```python
from build123d import *

# Parameters (mm, degrees)
EXTRUDE_1_DEPTH          = 5
CHAMFER_1_SIZE           = 10
CUT_EXTRUDE_1_DEPTH      = 61.279402969
CUT_EXTRUDE_1_DEPTH_BACK = 61.279402969
SKETCH_2_R               = 2.1
EXTRUDE_START            = 37
SKETCH_3_W               = 10
SKETCH_3_H               = 14.142135624
SKETCH_3_R               = 2.1
EXTRUDE_2_DEPTH          = 37
SKETCH_4_W               = 10
SKETCH_4_H               = 20
EXTRUDE_3_DEPTH          = 6
SKETCH_6_W               = 10
SKETCH_6_H               = 32
EXTRUDE_5_DEPTH          = 6
CUT_EXTRUDE_2_DEPTH      = 15
CUT_EXTRUDE_3_DEPTH      = 72.219678224
SKETCH_10_W              = 15
SKETCH_10_H              = 3.8
EXTRUDE_6_DEPTH          = 3
CHAMFER_2_SIZE           = 2
CHAMFER_3_SIZE           = 2
CHAMFER_4_SIZE           = 5
CHAMFER_5_SIZE           = 2
SKETCH_12_R              = 3.2
CUT_EXTRUDE_4_DEPTH      = 38
CUT_EXTRUDE_5_DEPTH      = 4


with BuildPart() as part:
    # 草图1 → 凸台-拉伸1 (new, symmetric)
    with BuildSketch(Plane.XY):
        Polygon((-10, 0), (33.5, 43.5), (38.5, 38.5), (0, 0), (38.5, -38.5), (33.5, -43.5), align=None)
    extrude(amount=EXTRUDE_1_DEPTH, both=True)

    # 倒角1
    chamfer_1_edges = [part.edges().sort_by_distance(p)[0] for p in [
        (-10, 0, 0),
        (0, 0, 0),
    ]]
    chamfer(chamfer_1_edges, length=CHAMFER_1_SIZE)

    # 草图2 → 切除-拉伸1 (cut, two sides: drawn at the far end of the back side and taken through both)
    with BuildSketch(Plane.ZY.offset(2.928932188).offset(-CUT_EXTRUDE_1_DEPTH_BACK)):
        with Locations(Location((0, 0, 0), (0, 0, 270))):
            Circle(SKETCH_2_R)
    extrude(amount=CUT_EXTRUDE_1_DEPTH + CUT_EXTRUDE_1_DEPTH_BACK, mode=Mode.SUBTRACT)

    # 草图3 → 凸台-拉伸2 (add)
    with BuildSketch(Plane.ZY.offset(2.928932188).offset(EXTRUDE_START)):
        Rectangle(SKETCH_3_W, SKETCH_3_H)
        with Locations(Location((0, 0, 0), (0, 0, 270))):
            Circle(SKETCH_3_R, mode=Mode.SUBTRACT)
    extrude(amount=-EXTRUDE_2_DEPTH)

    # 草图4 → 凸台-拉伸3 (add)
    with BuildSketch(Plane(origin=(38.5, 38.5, 0), x_dir=(0, 0, -1), z_dir=(0.7071067811865467, 0.7071067811865485, 0))):
        with Locations((-10, -2.928932188)):
            Rectangle(SKETCH_4_W, SKETCH_4_H)
    extrude_3 = extrude(amount=-EXTRUDE_3_DEPTH)

    # 草图6 → 凸台-拉伸5 (add)
    with BuildSketch(Plane(origin=(38.5, 38.5, 0), x_dir=(0, 0, -1), z_dir=(0.7071067811865467, 0.7071067811865485, 0))):
        with Locations((-10, 3.071067812)):
            Rectangle(SKETCH_6_W, SKETCH_6_H)
    extrude_5 = extrude(amount=-EXTRUDE_5_DEPTH)

    # 草图8 → 切除-拉伸2 (cut)
    with BuildSketch(Plane.XY.offset(15)):
        Polygon((21.549895398, 48.520458146), (44.177312396, 25.893041148), (46.864318164, 28.580046917), (24.236901166, 51.207463915), align=None)
    cut_extrude_2 = extrude(amount=-CUT_EXTRUDE_2_DEPTH, mode=Mode.SUBTRACT)

    # 草图9 → 切除-拉伸3 (cut, through all)
    with BuildSketch(Plane(origin=(0, 0, 5), x_dir=(-1, 0, 0), z_dir=(0, 0, -1))):
        Polygon((-32.722182541, 42.722182541), (-24.236901166, 51.207463915), (-25.014718626, 51.985281374), (-33.5, 43.5), align=None)
        Polygon((-21.549895398, 48.520458146), (-30.035176772, 40.035176772), (-29.257359313, 39.257359313), (-20.772077939, 47.742640687), align=None)
    cut_extrude_3 = extrude(amount=-CUT_EXTRUDE_3_DEPTH, mode=Mode.SUBTRACT)

    # 草图10 → 凸台-拉伸6 (add)
    with BuildSketch(Plane(origin=(-5, 5, 0), x_dir=(0, 0, 1), z_dir=(-0.7071067811865487, 0.7071067811865465, 0))):
        with Locations((7.5, 51.447222151)):
            Rectangle(SKETCH_10_W, SKETCH_10_H)
    extrude_6 = extrude(amount=-EXTRUDE_6_DEPTH)

    # 倒角2
    chamfer_2_edges = [part.edges().sort_by_distance(p)[0] for p in [
        (47.253226894, 28.968955647, 15),
        (31.378679656, 41.378679656, 15),
        (22.785533906, 22.785533906, -5),
        (43.788403666, 25.504132419, 5),
        (43.788403666, 25.504132419, 15),
        (15.285533906, 25.285533906, -5),
        (38.11109127, 38.11109127, 5),
        (47.253226894, 28.968955647, 5),
    ]]
    chamfer(chamfer_2_edges, length=CHAMFER_2_SIZE)

    # 镜向1: 凸台-拉伸3, 凸台-拉伸5, 切除-拉伸2, 切除-拉伸3, 凸台-拉伸6 across plane
    add(extrude_3.mirror(Plane.ZX))
    add(extrude_5.mirror(Plane.ZX))
    add(cut_extrude_2.mirror(Plane.ZX), mode=Mode.SUBTRACT)
    add(cut_extrude_3.mirror(Plane.ZX), mode=Mode.SUBTRACT)
    add(extrude_6.mirror(Plane.ZX))

    # 倒角3
    chamfer_3_edges = [part.edges().sort_by_distance(p)[0] for p in [
        (38.11109127, -38.11109127, 5),
        (15.285533906, -25.285533906, -5),
        (43.788403666, -25.504132419, 5),
        (43.788403666, -25.504132419, 15),
        (34.646268043, -34.646268043, 5),
        (47.253226894, -28.968955647, 5),
        (47.253226894, -28.968955647, 15),
        (31.378679656, -41.378679656, 15),
        (22.785533906, -22.785533906, -5),
    ]]
    chamfer(chamfer_3_edges, length=CHAMFER_3_SIZE)

    # 倒角4
    chamfer_4_edges = [part.edges().sort_by_distance(p)[0] for p in [
        (31.757359313, -36.757359313, 5),
        (31.757359313, 36.757359313, 5),
    ]]
    chamfer(chamfer_4_edges, length=CHAMFER_4_SIZE)

    # 倒角5
    chamfer_5_edges = [part.edges().sort_by_distance(p)[0] for p in [
        (-20.014718626, -7.071067812, -5),
        (-20.014718626, 7.071067812, -5),
        (-21.428932188, -7.071067812, 5),
        (-21.428932188, 7.071067812, 5),
    ]]
    chamfer(chamfer_5_edges, length=CHAMFER_5_SIZE)

    # 草图12 → 切除-拉伸4 (cut)
    with BuildSketch(Plane.ZY.offset(39.928932188)):
        with Locations(Location((0, 0, 0), (0, 0, 270))):
            Circle(SKETCH_12_R)
    extrude(amount=-CUT_EXTRUDE_4_DEPTH, mode=Mode.SUBTRACT)

    # 草图13 → 切除-拉伸5 (cut)
    with BuildSketch(Plane(origin=(7.071067812, 0, 0), x_dir=(0, 0, -1), z_dir=(1, 0, 0))):
        Polygon((2.107328483, -3.65), (4.214656965, 0), (2.107328483, 3.65), (-2.107328483, 3.65), (-4.214656965, 0), (-2.107328483, -3.65), align=None)
    extrude(amount=-CUT_EXTRUDE_5_DEPTH, mode=Mode.SUBTRACT)


solid = part.part
```
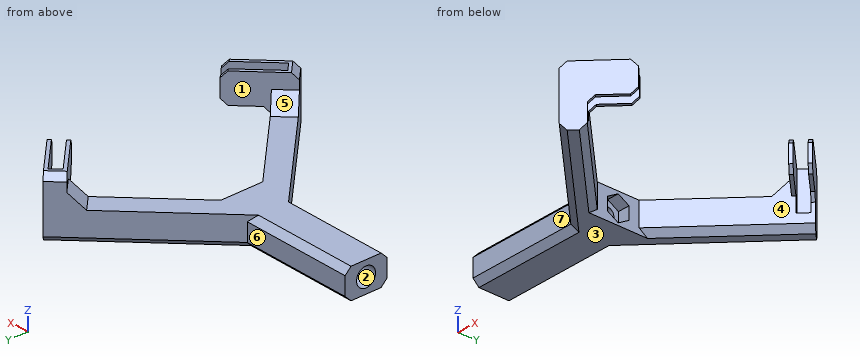
Verification items for the finished model (mm, model axes). Face numbers are marked on the shaded views. A direction names the side the tool comes from. Round coordinates to 2 decimals unless told otherwise and drop trailing zeros. Order: outer loops, then holes, each group sorted by start corner. A loop starts at its lowest first (then second) coordinate and runs counter-clockwise, first axis right, second up. Notation, with made-up numbers: (22, 63.25) - (57, 63.25) arc R31 ccw to (57, 101.25) - close; hole circle Ø8 at (68, 35.25). An arc over 180 degrees is marked (long way). Use CSV: the item, a comma, the result in double quotes. Start each with the question number.
1) Mould release check, pull along Y, two halves, no side actions. Record for the marked faces 4, 5, 6 and 7: +Y half, -Y half, draft (parallel to the pull), parting line (faces both ways), or undercut.
2) Section check D-D, the plane y = -15.5. Record the cut outline in (x, z), plus the area to 3 significant figures.
3) Go/stop test with flat-tipped pins: P1, Ø3.5, axis at y = -1, z = 2, coming from the +X side; P2, Ø1, axis at x = -19, y = 8.5, coming from the -Z side; P3, Ø5, axis at x = -26, z = -1, coming from the +Y side; P4, Ø10, axis at x = 11, z = -1.5, coming from the -Y side. Record where each tip stops, or that it passes through.
4) Section check B-B, the plane z = 8.25. Record the cut outline in (x, y).
5) Access from +Z, -Z, +X, -X, +Y, -Y to the whole of each face (thin tool, end or side, straight path). Record for the marked faces 1, 2 and 3.
6) Thickness scan on L1, parallel to Z at x = -17, y = 0; L2, parallel to Y at x = 38, z = 5.5; L3, parallel to Z at x = 1.75, y = 0. Record the ranges inside material, lowest first.
7) Section check C-C, the plane x = 13. Record the cut outline in (y, z), plus the area to 3 significant figures.
8) Section check A-A, the plane x = -28.5. Record the cut outline in (y, z).
Answers:
1,face 4,"undercut"
1,face 5,"undercut"
1,face 6,"+Y half"
1,face 7,"-Y half"
2,outline,"(5.5, -3) - (8.33, -5) - (12.67, -5) - (15.5, -3) - (15.5, 5) - (5.5, 5) - close"
2,area,"94.3 mm²"
3,P1,"stops at x = 7.07"
3,P2,"passes through"
3,P3,"stops at y = 7.07"
3,P4,"stops at y = -26"
4,outline,"(28.02, -38.02) - (33.5, -43.5) - (47.64, -29.36) - (46.86, -28.58) - (34.84, -40.6) - (32.16, -37.91) - (44.18, -25.89) - (43.4, -25.12) - (34.26, -34.26) - (33.02, -33.02) - close; (28.02, 38.02) - (33.02, 33.02) - (34.26, 34.26) - (43.4, 25.12) - (44.18, 25.89) - (32.16, 37.91) - (34.84, 40.6) - (46.86, 28.58) - (47.64, 29.36) - (33.5, 43.5) - close"
5,face 1,"+Z"
5,face 2,"-X"
5,face 3,"-Z, +X, -X, +Y, -Y"
6,L1,"z = -5 to -3.2, 3.2 to 5"
6,L2,"y = -39 to -37.44, -32.07 to -30.51, 30.51 to 32.07, 37.44 to 39"
6,L3,"z = -5 to -2.1, 2.1 to 5"
7,outline,"(-23, -3) - (-20.17, -5) - (-15.83, -5) - (-13, -3) - (-13, 5) - (-23, 5) - close; (13, -3) - (15.83, -5) - (20.17, -5) - (23, -3) - (23, 5) - (13, 5) - close"
7,area,"189 mm²"
8,outline,"(-7.07, -3) - (-5.07, -5) - (5.07, -5) - (7.07, -3) - (7.07, 3) - (5.07, 5) - (-5.07, 5) - (-7.07, 3) - close; hole circle Ø6.4 at (0, 0)"
